from build123d import *

# Parameters (mm, degrees)
SKETCH1_R             = 29.605080475
SKETCH1_R_2           = 23.004044152
BOSS_EXTRUDE1_DEPTH   = 19
BOSS_EXTRUDE1_2_DEPTH = 19
BOSS_EXTRUDE2_DEPTH   = 9
CUT_EXTRUDE1_DEPTH    = 4
FILLET1_R             = 1
FILLET2_R             = 40
FILLET4_R             = 22.5
BOSS_EXTRUDE3_START   = -35
BOSS_EXTRUDE3_DEPTH   = 35
CUT_EXTRUDE2_DEPTH    = 209.505251732
SKETCH6_R             = 4.5
CUT_EXTRUDE3_DEPTH    = 203.261290265


with BuildPart() as part:
    # Sketch1 → Boss-Extrude1 (new, symmetric)
    with BuildSketch(Plane.XY):
        Circle(SKETCH1_R)
        Circle(SKETCH1_R_2, mode=Mode.SUBTRACT)
    extrude(amount=BOSS_EXTRUDE1_DEPTH, both=True)


with BuildPart() as body_2:
    # Sketch1 → Boss-Extrude1 2 (new, symmetric)
    with BuildSketch(Plane.XY):
        with BuildLine():
            Line((-36, -201.2), (-27, -201.2))
            ThreePointArc((-27, -201.2), (0, -174.2), (27, -201.2))
            Line((27, -201.2), (36, -201.2))
            ThreePointArc((36, -201.2), (0, -165.2), (-36, -201.2))
        make_face()
    extrude(amount=BOSS_EXTRUDE1_2_DEPTH, both=True)

    # Sketch1<3> → Boss-Extrude2 (add, symmetric)
    with BuildSketch(Plane.XY):
        with BuildLine():
            ThreePointArc((10, -27.865046024), (5.075128567, -29.166828075), (0, -29.605080475))
            Line((0, -29.605080475), (0, -165.2))
            ThreePointArc((0, -165.2), (9.002752214, -166.343860619), (17.433399222, -169.702752635))
            Line((17.433399222, -169.702752635), (10, -27.865046024))
        make_face()
        with BuildLine():
            Line((0, -165.2), (0, -29.605080475))
            ThreePointArc((0, -29.605080475), (-5.075128567, -29.166828075), (-10, -27.865046024))
            Line((-10, -27.865046024), (-17.433399222, -169.702752635))
            ThreePointArc((-17.433399222, -169.702752635), (-9.002752214, -166.343860619), (0, -165.2))
        make_face()
    extrude(amount=BOSS_EXTRUDE2_DEPTH, both=True)

    # Sketch2 → Cut-Extrude1 (cut)
    with BuildSketch(Plane(origin=(0, 0, -9), x_dir=(-1, 0, 0), z_dir=(0, 0, -1))):
        with BuildLine():
            Line((-8, -138.611669698), (-8, -48.611669698))
            ThreePointArc((-8, -48.611669698), (0, -40.611669698), (8, -48.611669698))
            Line((8, -48.611669698), (8, -138.611669698))
            ThreePointArc((8, -138.611669698), (0, -146.611669698), (-8, -138.611669698))
        make_face()
    cut_extrude1 = extrude(amount=-CUT_EXTRUDE1_DEPTH, mode=Mode.SUBTRACT)

    # Mirror1: Cut-Extrude1 across plane
    add(cut_extrude1.mirror(Plane.XY), mode=Mode.SUBTRACT)

    # Fillet1
    fillet1_edges = [body_2.edges().sort_by_distance(p)[0] for p in [
        (0, -146.611669698, -5),
        (8, -93.611669698, -5),
        (0, -40.611669698, -5),
        (-8, -93.611669698, -5),
        (0, -146.611669698, 5),
        (-8, -93.611669698, 5),
        (0, -40.611669698, 5),
        (8, -93.611669698, 5),
    ]]
    fillet(fillet1_edges, radius=FILLET1_R)

    # Fillet2
    fillet2_edges = [body_2.edges().sort_by_distance(p)[0] for p in [
        (-17.433399222, -169.702752635, 0),
        (17.433399222, -169.702752635, 0),
    ]]
    fillet(fillet2_edges, radius=FILLET2_R)

    # Combine1: union part
    add(part.part)

    # Fillet4
    fillet4_edges = [body_2.edges().sort_by_distance(p)[0] for p in [
        (10, -27.865046024, 0),
        (-10, -27.865046024, 0),
    ]]
    fillet(fillet4_edges, radius=FILLET4_R)

    # Sketch3 → Boss-Extrude3 (add)
    with BuildSketch(Plane(origin=(0, -166.2, 0), x_dir=(1, 0, 0), z_dir=(0, 1, 0)).offset(BOSS_EXTRUDE3_START)):
        with BuildLine():
            Line((-38, 9), (38, 9))
            ThreePointArc((38, 9), (47, 0), (38, -9))
            Line((38, -9), (-38, -9))
            ThreePointArc((-38, -9), (-47, 0), (-38, 9))
        make_face()
    extrude(amount=BOSS_EXTRUDE3_DEPTH)

    # Sketch5 → Cut-Extrude2 (cut, through all)
    with BuildSketch(Plane.XY.offset(9)):
        with BuildLine():
            Line((-27, -201.2), (27, -201.2))
            ThreePointArc((27, -201.2), (0, -174.2), (-27, -201.2))
        make_face()
    extrude(amount=-CUT_EXTRUDE2_DEPTH, mode=Mode.SUBTRACT)

    # Sketch6 → Cut-Extrude3 (cut, through all)
    with BuildSketch(Plane(origin=(0, -166.2, 0), x_dir=(1, 0, 0), z_dir=(0, 1, 0))):
        with Locations(Location((-38, 0, 0), (0, 0, 270))):
            Circle(SKETCH6_R)
        with Locations(Location((38, 0, 0), (0, 0, 270))):
            Circle(SKETCH6_R)
    extrude(amount=-CUT_EXTRUDE3_DEPTH, mode=Mode.SUBTRACT)


solid = body_2.part
Geometry check sheet. Reference: the model listing, model coordinates, mm. A direction names the side the tool comes from. Coordinates: 2 decimals unless noted, no trailing zeros. Order: outer loops, then holes, each group sorted by start corner. A loop starts at its lowest first (then second) coordinate and runs counter-clockwise, first axis right, second up. Notation, with made-up numbers: (71, 51.5) - (94, 51.5) arc R10 ccw to (94, 59.5) - close; hole circle Ø8 at (37.25, 38.5). An arc over 180 degrees is marked (long way). One line per item, written item: value.
(1) Sectioned sample at C-C (z = 0). Enter the section's corners in (x, y).
Data:
outline: (-47, -201.2) - (-42.5, -201.2) - (-42.5, -166.2) - (-47, -166.2) - close; (-33.5, -201.2) - (-27, -201.2) arc R27 cw to (27, -201.2) - (33.5, -201.2) - (33.5, -166.2) - (19.75, -166.2) arc R40 cw to (16.53, -152.43) - (10.71, -41.36) arc R22.5 cw to (18.85, -22.83) arc R29.61 ccw (long way) to (-18.85, -22.83) arc R22.5 cw to (-10.71, -41.36) - (-16.53, -152.43) arc R40 cw to (-19.75, -166.2) - (-33.5, -166.2) - close; (42.5, -201.2) - (47, -201.2) - (47, -166.2) - (42.5, -166.2) - close; hole circle Ø46.01 at (0, 0)
(2) Access from +Z, -Z, +X, -X, +Y, -Y to the whole of each face (thin tool, end or side, straight path). Record for faces 4 (the face through (17.505, -159.363, 0.126)), 5 (the face through (0, -93, -5)), 6 (the face through (9, -126, 9)).
Data:
face 4: +Z, -Z, +X
face 5: -Z
face 6: +Z
(3) Sectioned sample at D-D (z = 15). Enter the section's corners in (x, y), and give its area (3 significant figures).
Data:
outline: (-36, -201.2) - (-27, -201.2) arc R27 cw to (27, -201.2) - (36, -201.2) arc R36 ccw to start; circle Ø59.21 at (0, 0); hole circle Ø46.01 at (0, 0)
area: 1,980 mm^2
(4) Sectioned sample at B-B (x = 0). Enter the section's corners in (y, z), and give its area (3 significant figures).
Data:
outline: (-174.2, -19) - (-165.2, -19) - (-165.2, -9) - (-146.61, -9) - (-146.61, -6) arc R1 cw to (-145.61, -5) - (-41.61, -5) arc R1 cw to (-40.61, -6) - (-40.61, -9) - (-29.61, -9) - (-29.61, -19) - (-23, -19) - (-23, 19) - (-29.61, 19) - (-29.61, 9) - (-40.61, 9) - (-40.61, 6) arc R1 cw to (-41.61, 5) - (-145.61, 5) arc R1 cw to (-146.61, 6) - (-146.61, 9) - (-165.2, 9) - (-165.2, 19) - (-174.2, 19) - close; (23, -19) - (29.61, -19) - (29.61, 19) - (23, 19) - close
area: 2,440 mm^2
(5) Thickness scan on probe 1 along Y at (x, z) = (0, 8.5); probe 2 along X at (y, z) = (-182, 0); probe 3 along Y at (x, z) = (0, 0). Record the ranges inside material, lowest first. Write a range as from..to.
Data:
probe 1: y = -174.2..-146.61, -40.61..-23, 23..29.61
probe 2: x = -47..-42.5, -33.5..-18.98, 18.98..33.5, 42.5..47
probe 3: y = -174.2..-23, 23..29.61
(6) Sectioned sample at A-A (y = 0). Enter the section's corners in (x, z), and give its area (3 significant figures).
Data:
outline: (-29.61, -19) - (-23, -19) - (-23, 19) - (-29.61, 19) - close; (23, -19) - (29.61, -19) - (29.61, 19) - (23, 19) - close
area: 502 mm^2
(7) Release check for a two-part mould opening along X. For faces 1 (the face through (-3.854, 29.353, 0.266)), 2 (the face through (-0.18, -146.61, 7.52)), 3 (the face through (-12.637, -30.991, -0.126)) record: +X half, -X half, draft (parallel to the pull), parting line (faces both ways), or undercut.
Data:
face 1: parting line
face 2: undercut
face 3: -X half
(8) Depth check by flat-ended pin: pin 1 Ø1 at (y, z) = (-18, 3) entering from -X; pin 2 Ø9 at (x, z) = (-28, -1) entering from +Y; pin 3 Ø1.5 at (y, z) = (-86.5, -7.5) entering from +X; pin 4 Ø10.5 at (x, z) = (38, 0) entering from -Y. Enter the tip coordinate at first touch or a pass-through.
Data:
pin 1: stops at x = -23.88
pin 2: stops at y = 18.01
pin 3: stops at x = 13.11
pin 4: stops at y = -201.2
